Job drawing, mm, ordinate dimensions from the low corner. One solid piece. A direction names the side the tool comes from. Round coordinates to 2 decimals unless told otherwise and drop trailing zeros. Write each loop counter-clockwise with the first axis right and the second up, starting at its lowest first coordinate (ties: lowest second). Pieces come first, ordered by that corner, then holes. Notation, with made-up numbers: (-5, 78) - (41, 78) arc R13 ccw to (41, 91) - close; hole circle Ø4 at (13.5, 21). An arc over 180 degrees is marked (long way). Write each question's results on one line, items separated by ' | '.
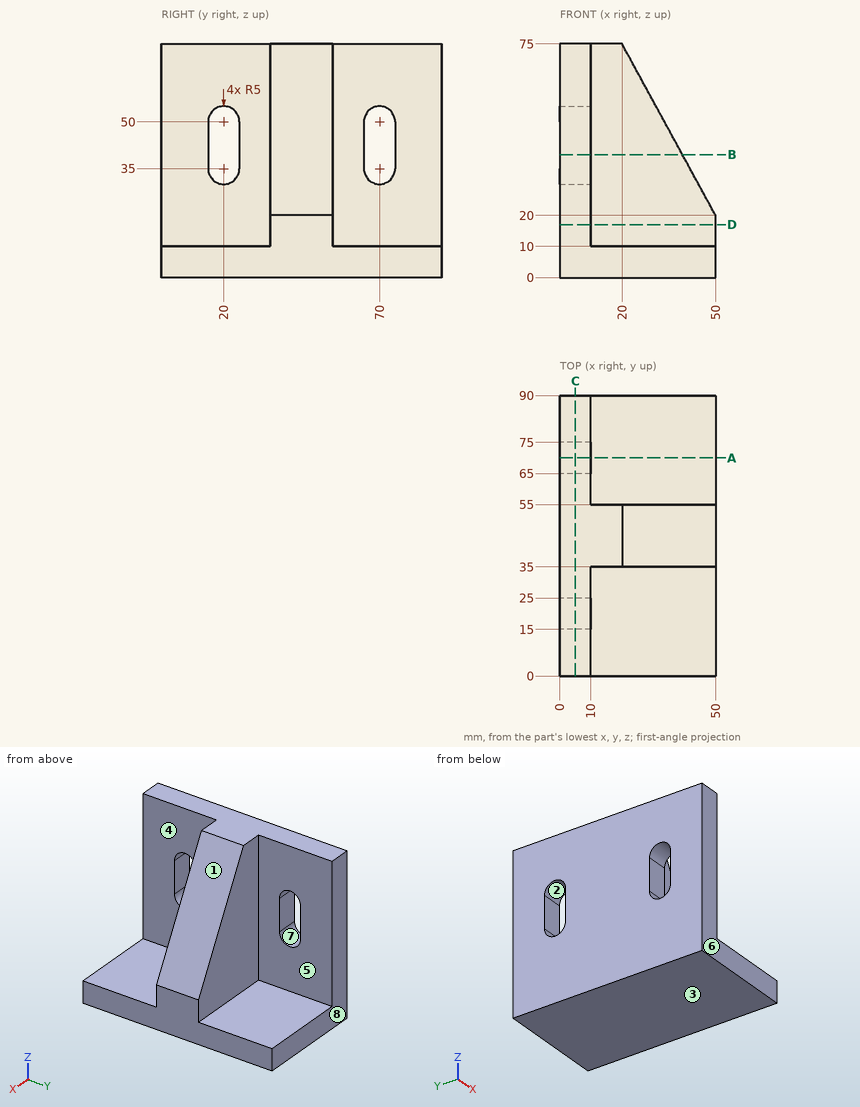
(1) Slice it at A-A, the plane y = 70. Write the cut outline in (x, z), and give its area (3 significant figures).
Worked answers:
outline: (0, 0) - (50, 0) - (50, 10) - (10, 10) - (10, 30) - (0, 30) - close; (0, 55) - (10, 55) - (10, 75) - (0, 75) - close | area: 900 mm2
(2) Slice it at D-D, the plane z = 17. Write the cut outline in (x, y), and give its area (3 significant figures).
Worked answers:
outline: (0, 0) - (10, 0) - (10, 35) - (50, 35) - (50, 55) - (10, 55) - (10, 90) - (0, 90) - close | area: 1,700 mm2
(3) Two-plate mould, pull along Y, no slides. Class the marked faces 6, 7 and 8: released by +Y, released by -Y, zero draft, split by the parting line, or undercut.
Worked answers:
face 6: released by -Y | face 7: undercut | face 8: released by +Y
(4) Drill centre lines: probe 1 along Y at (x, z) = (2, 53.5); probe 2 along Y at (x, z) = (8, 53); probe 3 along Y at (x, z) = (25, 38). Where is each one in solid material? Low to high. Write a range as [from, to].
Worked answers:
probe 1: y = [0, 16.43], [23.57, 66.43], [73.57, 90] | probe 2: y = [0, 16], [24, 66], [74, 90] | probe 3: y = [35, 55]
(5) Slice it at B-B, the plane z = 39.5. Write the cut outline in (x, y), and give its area (3 significant figures).
Worked answers:
outline: (0, 0) - (10, 0) - (10, 15) - (0, 15) - close; (0, 25) - (10, 25) - (10, 35) - (39.36, 35) - (39.36, 55) - (10, 55) - (10, 65) - (0, 65) - close; (0, 75) - (10, 75) - (10, 90) - (0, 90) - close | area: 1,290 mm2
(6) Slice it at C-C, the plane x = 5. Write the cut outline in (y, z), and give its area (3 significant figures).
Worked answers:
outline: (0, 0) - (90, 0) - (90, 75) - (0, 75) - close; hole (15, 35) arc R5 ccw to (25, 35) - (25, 50) arc R5 ccw to (15, 50) - close; hole (65, 35) arc R5 ccw to (75, 35) - (75, 50) arc R5 ccw to (65, 50) - close | area: 6,290 mm2
(7) Flat gauge pins, fed straight in: pin 1 Ø5 at (x, z) = (18, 66.5) entering from -Y; pin 2 Ø10.5 at (x, y) = (30, 80.5) entering from +Z; pin 3 Ø17.5 at (y, z) = (70, 58) entering from +X. Where does each tip first touch, or does it go through?
Worked answers:
pin 1: stops at y = 35 | pin 2: stops at z = 10 | pin 3: stops at x = 10
(8) Tool access for the marked faces 1, 2, 3, 4 and 5: list every direction of +Z, -Z, +X, -X, +Y, -Y with a clear straight run to the whole face (end or side of a thin tool).
Worked answers:
face 1: +Z, +X, +Y, -Y | face 2: +X, -X | face 3: -Z, +X, -X, +Y, -Y | face 4: +Z, +X, -Y | face 5: +Z, +X, +Y
